Autodesk Inventor part; units mm, degrees
ref_plane "YZ Plane" through (0, 0, 0) normal (1, 0, 0) x (0, 1, 0)
ref_plane "XZ Plane" through (0, 0, 0) normal (0, 1, 0) x (-1, 0, 0)
ref_plane "XY Plane" through (0, 0, 0) normal (0, 0, 1) x (1, 0, 0)
sketch "Sketch1" plane through (0, 0, 0) normal (0, 0, 1) x (1, 0, 0)
  line L0 (0, 0) -> (1397, 0)
  line L1 (1397, 0) -> (1397, 714.375)
  line L2 (1397, 714.375) -> (0, 714.375)
  line L3 (0, 714.375) -> (0, 0)
  dimension "d0" = 1397
  dimension "d1" = 714.375
extrude "Extrusion1" add sketch "Sketch1" along normal blind 15.875
sketch "Sketch10" plane through (0, 0, 15.875) normal (0, 0, 1) x (1, 0, 0)
  line L0 (0, 0) -> (1397, 0)
  line L1 (1397, 0) -> (1397, 714.375)
  line L2 (0, 714.375) -> (0, 0)
  line L3 (0, 540.5628) -> (44.45, 540.5628)
  line L4 (425.45, 0) -> (425.45, 44.45)
  line L5 (971.55, 0) -> (971.55, 44.45)
  line L6 (1397, 540.5628) -> (1352.55, 540.5628)
  dimension "d68" = 44.45
  dimension "d69" = 44.45
  dimension "d70" = 44.45
  dimension "d71" = 44.45
hole "Hole4" at (44.45, 540.5628, 15.875) at (425.45, 44.45, 15.875) at (971.55, 44.45, 15.875) at (1352.55, 540.5628, 15.875) direction (0, 0, -1) diameter 10.5918 depth 35.179 tip angle 118
sketch "Sketch15" plane through (0, 0, 15.875) normal (0, 0, 1) x (1, 0, 0)
  line L0 (0, 714.375) -> (0, 0)
  line L1 (0, 0) -> (88.9, 0)
  line L2 (0, 0) -> (1397, 0)
  line L3 (88.9, 0) -> (104.775, 0)
  line L4 (104.775, 0) -> (409.575, 0)
  line L5 (409.575, 0) -> (409.575, 409.575)
  line L6 (359.575, 359.575) -> (459.575, 359.575)
  line L7 (459.575, 359.575) -> (459.575, 459.575)
  line L8 (459.575, 459.575) -> (359.575, 459.575)
  line L9 (359.575, 459.575) -> (359.575, 359.575)
  line L10 (359.575, 359.575) -> (459.575, 459.575) construction
  line L11 (459.575, 359.575) -> (359.575, 459.575) construction
  dimension "d107" = 88.9
  dimension "d108" = 15.875
  dimension "d109" = 304.8
  dimension "d110" = 409.575
  dimension "d111" = 100
  dimension "d112" = 100
extrude "Extrusion6" cut sketch "Sketch15" against normal blind 15.875
properties part number "Half Ceiling Model 2"
Work out the finished part from the listing and answer in its coordinate system (mm). Give positions to 0.01 mm unless a question says otherwise; leave off trailing zeros. Loops run counter-clockwise (first coordinate to the right, second up) from the corner with the lowest first, then second, coordinate; pieces in that order, holes last. Notation, with made-up numbers: (81, 9) - (133, 9) arc R5 cw to (133, 13) - close; hole circle Ø3 at (5, -34.75). An arc over 180 degrees is marked (long way). Answer in a Markdown table with one row per item. Add a question column.
Q1. Consider line 1 along X through (y, z) = (44.45, 9.5); line 2 along Y through (x, z) = (425.45, 7.25) (3 decimals); line 3 along Y through (x, z) = (44.45, 10.25) (3 decimals). Determine where each line is inside the solid, lowest interval first.
Q2. This flat-tipped pin is pushed along its axis until it touches: P1, Ø8, axis at y = 410.5, z = 7.5, coming from the -X side. Where does it stop, or does it pass through?
Q3. The part is cut by section A-A (y = 442). Determine the outline of the cut face in (x, z) (3 decimals).
Solution:
| question | item | result |
|---|---|---|
| 1 | line 1 | x = 0 to 420.15, 430.75 to 966.25, 976.85 to 1397 |
| 1 | line 2 | y = 0 to 39.154, 49.746 to 359.575, 459.575 to 714.375 |
| 1 | line 3 | y = 0 to 535.267, 545.859 to 714.375 |
| 2 | P1 | stops at x = 0 |
| 3 | outline | (0, 0) - (359.575, 0) - (359.575, 15.875) - (0, 15.875) - close; (459.575, 0) - (1397, 0) - (1397, 15.875) - (459.575, 15.875) - close |
